Study the drawing (mm; zero at the part's minimum x, y, z) and answer. Give positions to 0.01 mm unless a question says otherwise; leave off trailing zeros. Loops run counter-clockwise (first coordinate to the right, second up) from the corner with the lowest first, then second, coordinate; pieces in that order, holes last. Notation, with made-up numbers: M 2,-4.5 L 41,-4.5 A13 ccw 41,7.5 Z; hole C -34,-32 d3. An arc over 180 degrees is marked long. Use one line per item in the form item = value. Start each with the question number.
1. The mould has two halves that part along X. Classify the marked faces 1, 2, 3 and 4: released by +X, released by -X, zero draft, split by the parting line, or undercut.
2. Each of these flat-tipped pins is pushed along its axis until it touches: pin 1 Ø12 at (x, y) = (116, 20) entering from +Z; pin 2 Ø3 at (x, y) = (50, 5) entering from -Z. Where does it stop, or does it pass through?
3. The part is cut by section B-B (y = 8). Write down the section's boundary in (x, z), and give its area (3 significant figures).
4. The part is cut by section C-C (x = 40). Write down the section's boundary in (y, z).
5. Straight lines are drawn through the part: line 1 (X direction, y = 29, z = 15.25); line 2 (Y direction, x = 28, z = 7.5); line 3 (Z direction, x = 55, y = 12). For each, find the intervals that lie inside material, in ascending order. Write a range as from..to.
6. The part is cut by section A-A (z = 9). Write down the section's boundary in (x, y), and give its area (3 significant figures).
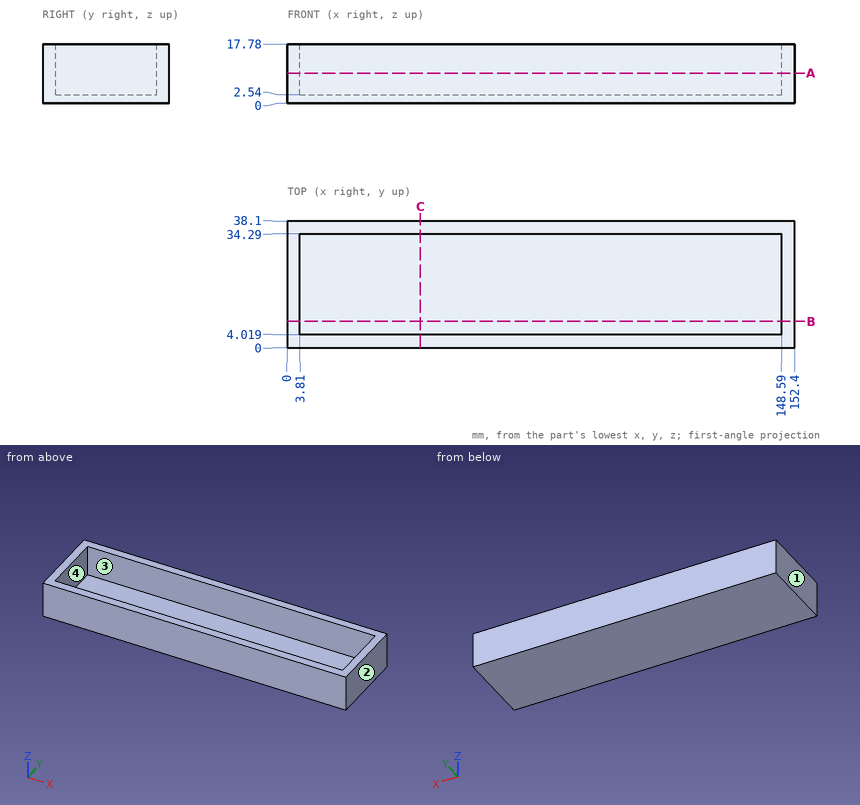
Derived:
q1.face_1 = released by -X
q1.face_2 = released by +X
q1.face_3 = undercut
q1.face_4 = undercut
q2.pin_1 = 2.54
q2.pin_2 = 0
q3.outline = M 0,0 L 152.4,0 L 152.4,17.78 L 148.59,17.78 L 148.59,2.54 L 3.81,2.54 L 3.81,17.78 L 0,17.78 Z
q3.area = 503 mm2
q4.outline = M 0,0 L 38.1,0 L 38.1,17.78 L 34.29,17.78 L 34.29,2.54 L 4.02,2.54 L 4.02,17.78 L 0,17.78 Z
q5.line_1 = 0..3.81, 148.59..152.4
q5.line_2 = 0..4.02, 34.29..38.1
q5.line_3 = 0..2.54
q6.outline = M 0,0 L 152.4,0 L 152.4,38.1 L 0,38.1 Z; hole M 3.81,4.02 L 148.59,4.02 L 148.59,34.29 L 3.81,34.29 Z
q6.area = 1,420 mm2
